from build123d import *

# Parameters (mm, degrees)
PRIMARY_START           = -87.9
SKETCH2_W               = 20.25
SKETCH2_H               = 60
SKETCH2_W_2             = 43.25
PRIMARY_EXTRUSION_DEPTH = 62.5
SKETCH3_R               = 3.175
CUT_EXTRUDE2_DEPTH      = 25.4
CUT_EXTRUDE3_START      = -62.5
SKETCH3_2_R             = 3.175
CUT_EXTRUDE3_DEPTH      = 6.35
CHAMFER1_SIZE           = 1.5875
CUT_EXTRUDE4_DEPTH      = 6.35
CUT_EXTRUDE5_DEPTH      = 153.4


with BuildPart() as part:
    # Sketch2 → Primary Extrusion (new body)
    with BuildSketch(Plane.XY.offset(PRIMARY_START)):
        with Locations((-135.5, 30)):
            Rectangle(SKETCH2_W, SKETCH2_H)
        with BuildLine():
            ThreePointArc((-132.325, 7), (-135.625, 3.7), (-138.925, 7))
            ThreePointArc((-138.925, 7), (-135.625, 10.3), (-132.325, 7))
        make_face(mode=Mode.SUBTRACT)
        with BuildLine():
            ThreePointArc((-132.325, 53), (-135.625, 49.7), (-138.925, 53))
            ThreePointArc((-138.925, 53), (-135.625, 56.3), (-132.325, 53))
        make_face(mode=Mode.SUBTRACT)
        with BuildLine():
            ThreePointArc((-138.925, 7), (-135.625, 3.7), (-132.325, 7))
            ThreePointArc((-132.325, 7), (-135.625, 10.3), (-138.925, 7))
        make_face()
        with BuildLine():
            ThreePointArc((-138.925, 53), (-135.625, 49.7), (-132.325, 53))
            ThreePointArc((-132.325, 53), (-135.625, 56.3), (-138.925, 53))
        make_face()
        with Locations((-167.25, 30)):
            Rectangle(SKETCH2_W_2, SKETCH2_H)
        Polygon((-145.625, 60), (-125.375, 60), (-125.375, 152.4), (-188.875, 152.4), (-188.875, 60), align=None)
    extrude(amount=PRIMARY_EXTRUSION_DEPTH)

    # Sketch3 → Cut-Extrude2 (cut)
    with BuildSketch(Plane.XY.offset(-25.4)):
        with Locations((-138.815833333, 47.3)):
            Circle(SKETCH3_R)
        with Locations((-138.815833333, 12.7)):
            Circle(SKETCH3_R)
        with Locations((93.595, 47.3)):
            Circle(SKETCH3_R)
        with Locations((131.655, 47.3)):
            Circle(SKETCH3_R)
        with Locations((131.655, 12.7)):
            Circle(SKETCH3_R)
        with Locations((93.595, 12.7)):
            Circle(SKETCH3_R)
        with Locations((-175.434166667, 47.3)):
            Circle(SKETCH3_R)
        with Locations((-175.434166667, 12.7)):
            Circle(SKETCH3_R)
    extrude(amount=-CUT_EXTRUDE2_DEPTH, mode=Mode.SUBTRACT)

    # Sketch3<2> → Cut-Extrude3 (cut)
    with BuildSketch(Plane.XY.offset(-25.4).offset(CUT_EXTRUDE3_START)):
        with Locations((-138.815833333, 47.3)):
            Circle(SKETCH3_2_R)
        with Locations((-138.815833333, 12.7)):
            Circle(SKETCH3_2_R)
    extrude(amount=CUT_EXTRUDE3_DEPTH, mode=Mode.SUBTRACT)

    # Chamfer1
    chamfer1_edges = [part.edges().sort_by_distance(p)[0] for p in [
        (-157.125, 0, -25.4),
        (-125.375, 76.2, -25.4),
        (-188.875, 76.2, -25.4),
    ]]
    chamfer(chamfer1_edges, length=CHAMFER1_SIZE)

    # Sketch4 → Cut-Extrude4 (cut)
    with BuildSketch(Plane.XZ):
        with BuildLine():
            ThreePointArc((-153.189971157, -75.335028843), (-150.439971157, -78.085028843), (-147.689971157, -75.335028843))
            ThreePointArc((-147.689971157, -75.335028843), (-150.439971157, -72.585028843), (-153.189971157, -75.335028843))
        make_face()
        with BuildLine():
            ThreePointArc((-166.625, -80.9), (-163.875, -83.65), (-161.125, -80.9))
            ThreePointArc((-161.125, -80.9), (-163.875, -78.15), (-166.625, -80.9))
        make_face()
        with BuildLine():
            ThreePointArc((-180.060028843, -75.335028843), (-177.310028843, -78.085028843), (-174.560028843, -75.335028843))
            ThreePointArc((-174.560028843, -75.335028843), (-177.310028843, -72.585028843), (-180.060028843, -75.335028843))
        make_face()
        with BuildLine():
            ThreePointArc((-153.189971157, -48.464971157), (-150.439971157, -51.214971157), (-147.689971157, -48.464971157))
            ThreePointArc((-147.689971157, -48.464971157), (-150.439971157, -45.714971157), (-153.189971157, -48.464971157))
        make_face()
        with BuildLine():
            ThreePointArc((-166.625, -42.9), (-163.875, -45.65), (-161.125, -42.9))
            ThreePointArc((-161.125, -42.9), (-163.875, -40.15), (-166.625, -42.9))
        make_face()
        with BuildLine():
            ThreePointArc((-180.060028843, -48.464971157), (-177.310028843, -51.214971157), (-174.560028843, -48.464971157))
            ThreePointArc((-174.560028843, -48.464971157), (-177.310028843, -45.714971157), (-180.060028843, -48.464971157))
        make_face()
    extrude(amount=-CUT_EXTRUDE4_DEPTH, mode=Mode.SUBTRACT)

    # Sketch4<4> → Cut-Extrude5 (cut, through all)
    with BuildSketch(Plane.XZ):
        with BuildLine():
            ThreePointArc((-171.875, -61.9), (-163.875, -69.9), (-155.875, -61.9))
            ThreePointArc((-155.875, -61.9), (-163.875, -53.9), (-171.875, -61.9))
        make_face()
    extrude(amount=-CUT_EXTRUDE5_DEPTH, mode=Mode.SUBTRACT)


solid = part.part
Check sheet for the modelled part. Datum: model origin and axes. Units: mm. A direction names the side the tool comes from. Give positions to 0.01 mm unless a question says otherwise; leave off trailing zeros. Order: outer loops, then holes, each group sorted by start corner. A loop starts at its lowest first (then second) coordinate and runs counter-clockwise, first axis right, second up. Notation, with made-up numbers: M 27.5,-7 L 83.5,-7 A29 cw 83.5,21 Z; hole C 32.25,29.25 d1. An arc over 180 degrees is marked long. Answer as CSV lines item,"result". Start each with the question number.
Item 1: Mould release check, pull along Y, two halves, no side actions. Record for faces 1 (the face through (-169.77, 75.13, -56.49)), 2 (the face through (-177, 6.35, -48)), 3 (the face through (-172.501, 11.484, -37.922)): +Y half, -Y half, draft (parallel to the pull), parting line (faces both ways), or undercut.
Item 2: Cross-section at C-C on z = -42.9. Enter the section's corners in (x, y) (3 decimals), plus the area to 3 significant figures.
Item 3: Cross-section at D-D on x = -137.5. Enter the section's corners in (y, z).
Item 4: Tool access check on faces 4 (the face through (-148.962, 3.131, -73.016)), 5 (the face through (-139, 13, -50.8)), 6 (the face through (-139, 47, -81.55)), 7 (the face through (-158, 77, -87.9)). Record the directions out of +Z, -Z, +X, -X, +Y, -Y that give a thin tool (end or side, any length) a straight path to the whole face; none if there is none.
Item 5: Cross-section at A-A on z = -61.9. Enter the section's corners in (x, y) (3 decimals).
Item 6: Gauge pin test, flat ends, axial feed: P1, Ø5, axis at x = -150.44, z = -48.46, coming from the -Y side; P2, Ø5, axis at x = -138.82, y = 47.3, coming from the +Z side; P3, Ø5, axis at x = -138.82, y = 47.3, coming from the -Z side. Record the tip position at first contact, or that the pin passes through.
Item 7: Thickness scan on line 1 (Y direction, x = -175.5, z = -48); line 2 (X direction, y = 11, z = -32.5) (3 decimals); line 3 (X direction, y = 47, z = -84) (3 decimals). Record the ranges inside material, lowest first. Write a range as [from, to].
Established:
1,face 1,"draft"
1,face 2,"-Y half"
1,face 3,"undercut"
2,outline,"M -188.875,0 L -166.625,0 L -166.625,6.35 L -161.125,6.35 L -161.125,0 L -125.375,0 L -125.375,152.4 L -188.875,152.4 Z; hole C -175.434,12.7 d6.35; hole C -175.434,47.3 d6.35; hole C -138.816,12.7 d6.35; hole C -138.816,47.3 d6.35"
2,area,"9,520 mm^2"
3,outline,"M 0,-87.9 L 9.81,-87.9 L 9.81,-81.55 L 15.59,-81.55 L 15.59,-87.9 L 44.41,-87.9 L 44.41,-81.55 L 50.19,-81.55 L 50.19,-87.9 L 152.4,-87.9 L 152.4,-25.4 L 50.19,-25.4 L 50.19,-50.8 L 44.41,-50.8 L 44.41,-25.4 L 15.59,-25.4 L 15.59,-50.8 L 9.81,-50.8 L 9.81,-25.4 L 1.59,-25.4 L 0,-26.99 Z"
4,face 4,"-Y"
4,face 5,"+Z"
4,face 6,"-Z"
4,face 7,"-Z, +X, -X, +Y, -Y"
5,outline,"M -188.875,0 L -171.875,0 L -171.875,152.4 L -188.875,152.4 Z; M -155.875,0 L -125.375,0 L -125.375,152.4 L -155.875,152.4 Z"
6,P1,"stops at y = 6.35"
6,P2,"stops at z = -50.8"
6,P3,"stops at z = -81.55"
7,line 1,"y = [6.35, 9.53], [15.87, 44.13], [50.47, 152.4]"
7,line 2,"x = [-188.875, -178.116], [-172.753, -141.497], [-136.134, -125.375]"
7,line 3,"x = [-188.875, -141.977], [-135.655, -125.375]"
